Work out the finished part from the listing and answer in its coordinate system (mm). A direction names the side the tool comes from. Coordinates: 2 decimals unless noted, no trailing zeros. Loops run counter-clockwise (first coordinate to the right, second up) from the corner with the lowest first, then second, coordinate; pieces in that order, holes last.
```python
from build123d import *

# Parameters (mm, degrees)
BOSS_EXTRUDE1_DEPTH = 3
SKETCH2_R           = 2.1
SKETCH2_R_2         = 1.5
CUT_EXTRUDE1_DEPTH  = 4


with BuildPart() as part:
    # Sketch1 → Boss-Extrude1 (new body)
    with BuildSketch(Plane(origin=(0, 0, 0), x_dir=(1, 0, 0), z_dir=(0, 1, 0))):
        with BuildLine():
            Line((-12.5, 42.656212912), (-12.447999296, 42.570796715))
            ThreePointArc((-12.447999296, 42.570796715), (-10.623582733, 38.374834362), (-10, 33.842093422))
            Line((-10, 33.842093422), (-10, 16.408985467))
            ThreePointArc((-10, 16.408985467), (-15.066740521, 2.488230295), (-27.896177884, -4.91884882))
            Line((-27.896177884, -4.91884882), (-30.873723057, -5.44387037))
            ThreePointArc((-30.873723057, -5.44387037), (0, -31.35), (30.873723057, -5.44387037))
            Line((30.873723057, -5.44387037), (27.896177884, -4.91884882))
            ThreePointArc((27.896177884, -4.91884882), (15.066740521, 2.488230295), (10, 16.408985467))
            Line((10, 16.408985467), (10, 33.842093422))
            ThreePointArc((10, 33.842093422), (10.623582733, 38.374834362), (12.447999296, 42.570796715))
            Line((12.447999296, 42.570796715), (12.5, 42.656212912))
            ThreePointArc((12.5, 42.656212912), (0, 44.45), (-12.5, 42.656212912))
        make_face()
    extrude(amount=BOSS_EXTRUDE1_DEPTH)

    # Sketch2 → Cut-Extrude1 (cut, through all)
    with BuildSketch(Plane(origin=(0, 3, 0), x_dir=(1, 0, 0), z_dir=(0, 1, 0))):
        with Locations((0, 0.014087551)):
            Circle(SKETCH2_R)
        with Locations((10, 0.014087551)):
            Circle(SKETCH2_R_2)
        with Locations((0, 10.014087551)):
            Circle(SKETCH2_R_2)
        with Locations((-10, 0.014087551)):
            Circle(SKETCH2_R_2)
        with Locations((0, -9.985912449)):
            Circle(SKETCH2_R_2)
    extrude(amount=-CUT_EXTRUDE1_DEPTH, mode=Mode.SUBTRACT)


solid = part.part
```
1. Each of these flat-tipped pins is pushed along its axis until it touches: P1, Ø1, axis at y = 2, z = -14, coming from the +X side; P2, Ø2.5, axis at x = 0, z = 9.99, coming from the -Y side; P3, Ø0.9, axis at y = 1.5, z = -25.5, coming from the +X side. Where does it stop, or does it pass through?
2. A cutting plane is placed at B-B, the plane y = 0.55. Give the vertices of the cut face in (x, z).
3. Determine the mould class of faces 4 (the cylindrical face through (-14.93, 1.48, -2.65)), 5 (the cylindrical face through (-0.33, 1.52, 11.45)), 6 (the cylindrical face through (-0.613, 1.479, 31.344)) for opening direction X: released by +X, released by -X, zero draft, split by the parting line, or undercut.
4. A cutting plane is placed at A-A, the plane x = 0. Give the vertices of the cut face in (y, z), then the cut area to 3 significant figures.
5. A cutting plane is placed at C-C, the plane z = -22. Give the vertices of the cut face in (x, y).
6. A cutting plane is placed at D-D, the plane x = 21.5. Give the vertices of the cut face in (y, z).
7. For faces 1 (the cylindrical face through (-10.64, 1.48, -38.44)), 2 (the cylindrical face through (0.18, 1.48, -44.45)), 3 (the flat face through (10, 1, -25)), determine the directions among +Z, -Z, +X, -X, +Y, -Y from which every point of the face is accessible in a straight line to the end or side of a thin tool.
8. Straight lines are drawn through the part: probe 1 along X at (y, z) = (2.35, -0.5); probe 2 along X at (y, z) = (0.8, -16.5); probe 3 along Z at (x, y) = (9, 1.4). For each, find the intervals that lie inside material, in ascending order.
Answers below:
1. P1: stops at x = 10.2
1. P2: passes through
1. P3: stops at x = 10
2. outline: (-30.87, 5.44) - (-27.9, 4.92) arc R21.66 cw to (-10, -16.41) - (-10, -33.84) arc R16.79 cw to (-12.45, -42.57) - (-12.5, -42.66) arc R44.45 ccw to (12.5, -42.66) - (12.45, -42.57) arc R16.79 cw to (10, -33.84) - (10, -16.41) arc R21.66 cw to (27.9, 4.92) - (30.87, 5.44) arc R31.35 ccw to start; hole circle Ø3 at (-10, -0.01); hole circle Ø4.2 at (0, -0.01); hole circle Ø3 at (0, -10.01); hole circle Ø3 at (0, 9.99); hole circle Ø3 at (10, -0.01)
3. face 4: released by -X
3. face 5: undercut
3. face 6: split by the parting line
4. outline: (0, -44.45) - (3, -44.45) - (3, -11.51) - (0, -11.51) - close; (0, -8.51) - (3, -8.51) - (3, -2.11) - (0, -2.11) - close; (0, 2.09) - (3, 2.09) - (3, 8.49) - (0, 8.49) - close; (0, 11.49) - (3, 11.49) - (3, 31.35) - (0, 31.35) - close
4. area: 197 mm2
5. outline: (-10, 0) - (10, 0) - (10, 3) - (-10, 3) - close
6. outline: (0, 2.72) - (3, 2.72) - (3, 22.82) - (0, 22.82) - close
7. face 1: -X, +Y, -Y
7. face 2: -Z, +Y, -Y
7. face 3: +X, +Y, -Y
8. probe 1: x = -16.96 to -11.42, -8.58 to -2.04, 2.04 to 8.58, 11.42 to 16.96
8. probe 2: x = -10 to 10
8. probe 3: z = -43.53 to -1.13, 1.1 to 30.03
